from build123d import *

# Parameters (mm, degrees)
BOSS_EXTRUDE5_DEPTH = 50
BOSS_EXTRUDE6_START = 20
BOSS_EXTRUDE6_DEPTH = 30
SKETCH1_5_R         = 10
BOSS_EXTRUDE7_DEPTH = 30
BOSS_EXTRUDE8_START = 20
BOSS_EXTRUDE8_DEPTH = 10


with BuildPart() as part:
    # Sketch1 → Boss-Extrude5 (new body)
    with BuildSketch(Plane(origin=(0, 0, 0), x_dir=(1, 0, 0), z_dir=(0, 1, 0))):
        with BuildLine():
            Line((-14, -5.385164807), (-14, -17.613914954))
            ThreePointArc((-14, -17.613914954), (0, -22.5), (14, -17.613914954))
            Line((14, -17.613914954), (14, -5.385164807))
            ThreePointArc((14, -5.385164807), (0, -15), (-14, -5.385164807))
        make_face()
        with BuildLine():
            ThreePointArc((14, 17.613914954), (0, 22.5), (-14, 17.613914954))
            Line((-14, 17.613914954), (-14, 5.385164807))
            ThreePointArc((-14, 5.385164807), (0, 15), (14, 5.385164807))
            Line((14, 5.385164807), (14, 17.613914954))
        make_face()
    extrude(amount=BOSS_EXTRUDE5_DEPTH)

    # Sketch1_4 → Boss-Extrude6 (add)
    with BuildSketch(Plane(origin=(0, 0, 0), x_dir=(1, 0, 0), z_dir=(0, 1, 0)).offset(BOSS_EXTRUDE6_START)):
        with BuildLine():
            Line((14, -5.385164807), (14, -17.613914954))
            ThreePointArc((14, -17.613914954), (20.263884129, -9.778803608), (22.5, 0))
            ThreePointArc((22.5, 0), (20.263884129, 9.778803608), (14, 17.613914954))
            Line((14, 17.613914954), (14, 5.385164807))
            ThreePointArc((14, 5.385164807), (14.747881204, 2.738612788), (15, 0))
            ThreePointArc((15, 0), (14.747881204, -2.738612788), (14, -5.385164807))
        make_face()
        with BuildLine():
            ThreePointArc((-14, 17.613914954), (-22.5, 0), (-14, -17.613914954))
            Line((-14, -17.613914954), (-14, -5.385164807))
            ThreePointArc((-14, -5.385164807), (-15, 0), (-14, 5.385164807))
            Line((-14, 5.385164807), (-14, 17.613914954))
        make_face()
    extrude(amount=BOSS_EXTRUDE6_DEPTH)

    # Sketch1_5 → Boss-Extrude7 (add)
    with BuildSketch(Plane(origin=(0, 0, 0), x_dir=(1, 0, 0), z_dir=(0, 1, 0))):
        with BuildLine():
            Line((-14, 5.385164807), (-14, -5.385164807))
            ThreePointArc((-14, -5.385164807), (0, -15), (14, -5.385164807))
            Line((14, -5.385164807), (14, 5.385164807))
            ThreePointArc((14, 5.385164807), (0, 15), (-14, 5.385164807))
        make_face()
        with Locations(Location((0, 0, 0), (0, 0, 270))):
            Circle(SKETCH1_5_R, mode=Mode.SUBTRACT)
    extrude(amount=BOSS_EXTRUDE7_DEPTH)

    # Sketch1_6 → Boss-Extrude8 (add)
    with BuildSketch(Plane(origin=(0, 0, 0), x_dir=(1, 0, 0), z_dir=(0, 1, 0)).offset(BOSS_EXTRUDE8_START)):
        with BuildLine():
            Line((14, 5.385164807), (14, -5.385164807))
            ThreePointArc((14, -5.385164807), (14.747881204, -2.738612788), (15, 0))
            ThreePointArc((15, 0), (14.747881204, 2.738612788), (14, 5.385164807))
        make_face()
        with BuildLine():
            ThreePointArc((-14, 5.385164807), (-15, 0), (-14, -5.385164807))
            Line((-14, -5.385164807), (-14, 5.385164807))
        make_face()
    extrude(amount=BOSS_EXTRUDE8_DEPTH)


solid = part.part
Source: CAD feature listing. Evaluate the final solid. Frame: model axes, mm. A direction names the side the tool comes from. Coordinates: 2 decimals unless noted, no trailing zeros. Write each loop counter-clockwise with the first axis right and the second up, starting at its lowest first coordinate (ties: lowest second). Pieces come first, ordered by that corner, then holes. Notation, with made-up numbers: M 0,-20 L 41,-20 A11 ccw 41,-12 Z; hole C -28.75,0 d3. An arc over 180 degrees is marked long. Use a Markdown table: item, result.
1) Section A-A, the plane y = 39.5. Output: boundary loops of the cut face in (x, z), then the cut area to 3 significant figures.
Conclusion:
| item | result |
|---|---|
| outline | C 0,0 d45; hole C 0,0 d30 |
| area | 884 mm^2 |
2) Mould query, pull axis Z, two halves, no side actions, for faces 1 (the flat face through (-14, 10, 0)), 2 (the flat face through (3, 30, 10)). Classes: pulls with the +Z half, pulls with the -Z half, needs draft (parallel to the pull), parting line crosses it, or undercut.
Conclusion:
| item | result |
|---|---|
| face 1 | needs draft |
| face 2 | undercut |
3) Ray query, L1, parallel to X at y = 15, z = 0; L2, parallel to X at y = 35.5, z = 4; L3, parallel to X at y = 15, z = -14.5. Return the intervals inside material, ascending.
Conclusion:
| item | result |
|---|---|
| L1 | x = -14 to -10, 10 to 14 |
| L2 | x = -22.14 to -14.46, 14.46 to 22.14 |
| L3 | x = -14 to 14 |
4) Section D-D, the plane x = -4.5. Output: boundary loops of the cut face in (y, z).
Conclusion:
| item | result |
|---|---|
| outline | M 0,-22.05 L 50,-22.05 L 50,-14.31 L 30,-14.31 L 30,-8.93 L 0,-8.93 Z; M 0,8.93 L 30,8.93 L 30,14.31 L 50,14.31 L 50,22.05 L 0,22.05 Z |
5) First-contact query: pin 1 Ø4 at (x, z) = (-20, 5.5) entering from -Y; pin 2 Ø8 at (y, z) = (9.5, -2.5) entering from +X; pin 3 Ø5 at (x, y) = (5.5, 6) entering from -Z; pin 4 Ø18 at (x, z) = (0, 0) entering from -Y. Flat tips, straight axial feed; report the tip coordinate or a pass-through.
Conclusion:
| item | result |
|---|---|
| pin 1 | stops at y = 20 |
| pin 2 | stops at x = 14 |
| pin 3 | stops at z = -22.3 |
| pin 4 | passes through |
6) Section B-B, the plane x = 0. Output: boundary loops of the cut face in (y, z), then the cut area to 3 significant figures.
Conclusion:
| item | result |
|---|---|
| outline | M 0,-22.5 L 50,-22.5 L 50,-15 L 30,-15 L 30,-10 L 0,-10 Z; M 0,10 L 30,10 L 30,15 L 50,15 L 50,22.5 L 0,22.5 Z |
| area | 1,050 mm^2 |
7) Reachability of faces 3 (the flat face through (14, 10, 0)), 4 (the flat face through (-0.2, 0, -10.3)), 5 (the flat face through (-17, 20, 0)) from +Z, -Z, +X, -X, +Y, -Y: full face, straight path, thin tool, end or side. Return the list, or none.
Conclusion:
| item | result |
|---|---|
| face 3 | +Z, -Z, +X, -Y |
| face 4 | +Z, -Z, +X, -X, -Y |
| face 5 | +Z, -Z, -X, -Y |
8) Section C-C, the plane z = -14. Output: boundary loops of the cut face in (x, y).
Conclusion:
| item | result |
|---|---|
| outline | M -17.61,20 L -14,20 L -14,0 L 14,0 L 14,20 L 17.61,20 L 17.61,50 L 5.39,50 L 5.39,30 L -5.39,30 L -5.39,50 L -17.61,50 Z |
